Autodesk Inventor part; units mm, degrees
ref_plane "YZ Plane" through (0, 0, 0) normal (1, 0, 0) x (0, 1, 0)
ref_plane "XZ Plane" through (0, 0, 0) normal (0, 1, 0) x (-1, 0, 0)
ref_plane "XY Plane" through (0, 0, 0) normal (0, 0, 1) x (1, 0, 0)
sketch "Sketch1" plane through (0, 0, 0) normal (0, 0, 1) x (1, 0, 0)
  circle A0 centre (49.25, 5.6396) radius 1.625
  circle A1 centre (69.7498, 17.4021) radius 1.6
  circle A2 centre (49.25, 5.6396) radius 2.625
  circle A3 centre (69.7498, 17.4021) radius 2.6
  line L0 (50.4505, 7.9739) -> (67.3082, 18.2959)
  line L1 (51.875, 5.6396) -> (68.5894, 15.0754)
  point P0 (0, 0)
  dimension "d0" = 1
  dimension "d1" = 1
extrude "Extrusion1" add sketch "Sketch1" along normal mid plane 3.5
properties part number "palanca_proxima_media"
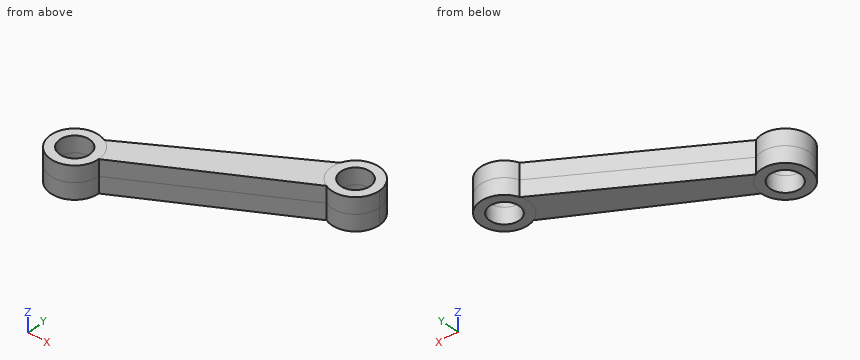
Work out the finished part from the listing and answer in its coordinate system (mm). Round coordinates to 2 decimals unless told otherwise and drop trailing zeros. Write each loop counter-clockwise with the first axis right and the second up, starting at its lowest first coordinate (ties: lowest second). Pieces come first, ordered by that corner, then holes. Notation, with made-up numbers: (-24, 17) - (2, 17) arc R17 cw to (2, 27) - close; hole circle Ø3 at (39.5, 41.5). An arc over 180 degrees is marked (long way). Return JSON: item names as keys, results as strings. Group by question number.
Q1. The part is cut by section A-A on x = 49.25. Write down the section's boundary in (y, z), then the cut area to 3 significant figures.
Q2. The part is cut by section B-B on y = 17.75. Write down the section's boundary in (x, z), then the cut area to 3 significant figures.
Q3. The part is cut by section C-C on z = 0.3. Count the separate pieces of the cut face and the enclosed holes in it, then the cut area to 3 significant figures.
Q4. Each of these flat-tipped pins is pushed along its axis until it touches: pin 1 Ø3 at (x, y) = (49.25, 5.64) entering from -Z; pin 2 Ø1.5 at (y, z) = (13, -0.5) entering from -X; pin 3 Ø1 at (x, z) = (52, 1) entering from -Y; pin 4 Ø1 at (y, z) = (15.5, 1.5) entering from -X. Where does it stop, or does it pass through?
Q5. The part is cut by section D-D on x = 65. Write down the section's boundary in (y, z), then the cut area to 3 significant figures.
Q6. Find the intervals of material crossed by L1, parallel to Y at x = 49.25, z = -1.3; L2, parallel to X at y = 5, z = -1.4; L3, parallel to X at y = 16.5, z = 0.15, in increasing order.
Solved:
{
 "1": {"outline": "(3.01, -1.75) - (4.01, -1.75) - (4.01, 1.75) - (3.01, 1.75) - close; (7.26, -1.75) - (8.26, -1.75) - (8.26, 1.75) - (7.26, 1.75) - close", "area": "7.00 mm²"},
 "2": {"outline": "(66.42, -1.75) - (68.19, -1.75) - (68.19, 1.75) - (66.42, 1.75) - close; (71.31, -1.75) - (72.33, -1.75) - (72.33, 1.75) - (71.31, 1.75) - close", "area": "9.75 mm²"},
 "3": {"separate pieces": "1", "enclosed holes": "2", "area": "84.2 mm²"},
 "4": {"pin 1": "through", "pin 2": "x = 57.43", "pin 3": "y = 4.29", "pin 4": "x = 61.93"},
 "5": {"outline": "(13.05, -1.75) - (16.88, -1.75) - (16.88, 1.75) - (13.05, 1.75) - close", "area": "13.4 mm²"},
 "6": {"L1": "3.01 to 4.01, 7.26 to 8.26", "L2": "46.7 to 47.76, 50.74 to 51.8", "L3": "64.38 to 68.43, 71.07 to 72.19"}
}
